Could you check a few things on this model? Use its own coordinates, in mm. Face numbers are marked on the shaded views. Round coordinates to 2 decimals unless told otherwise and drop trailing zeros. Loops run counter-clockwise (first coordinate to the right, second up) from the corner with the lowest first, then second, coordinate; pieces in that order, holes last. Notation, with made-up numbers: (13, 9.25) - (52, 9.25) arc R12 ccw to (52, 30.25) - close; hole circle Ø10 at (-26, -30.75). An arc over 180 degrees is marked (long way). Answer as CSV lines item,"result". Start each with the question number.
1) Suppose I cut it at C-C, the plane y = -25. Write out the boundary of the cut face in (x, z), then the cut area to 3 significant figures.
2) Suppose I cut it at A-A, the plane z = 7. Write out the boundary of the cut face in (x, y).
3) We'd pull the mould along X, two halves only. Please class the marked faces 1, 2, 3 and 4: pulls with the +X half, pulls with the -X half, needs draft (parallel to the pull), parting line crosses it, or undercut.
4) I'm going to push a flat-ended pin straight in: pin 1 Ø6 at (y, z) = (-19, 21.5) entering from -X. Where does the tip first touch, or does it pass through?
5) Suppose I cut it at D-D, the plane x = 16.25. Write out the boundary of the cut face in (y, z).
6) Please list where these lines run through material, in increasing order: line 1 along X through (y, z) = (-26.5, 10.25); line 2 along Z through (x, y) = (10.5, -19); line 3 along Y through (x, z) = (17.75, 10.25).
7) Suppose I cut it at B-B, the plane z = 17.25. Write out the boundary of the cut face in (x, y), then the cut area to 3 significant figures.
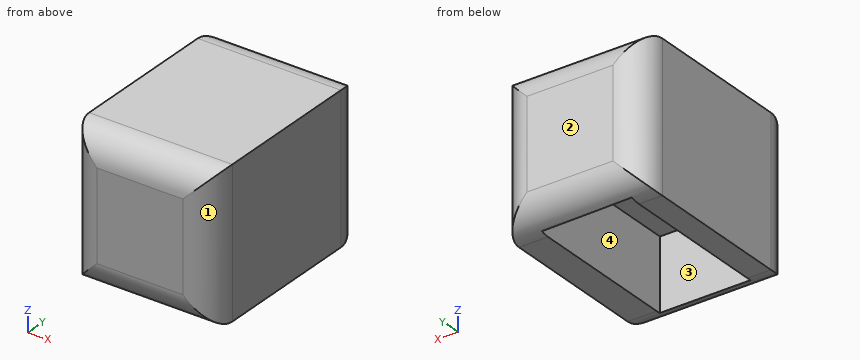
```python
from build123d import *

# Parameters (mm, degrees)
F0_W        = 36.6208925843
F0_H        = 25.9851198643
F1_DEPTH    = 25.4
F3_DEPTH    = 12.7
F4_DEPTH    = 12.7
F5_T1_DEPTH = 50.8
F5_T3_DEPTH = 51.3851198643
F6_T1_DEPTH = 50.8
F6_T3_DEPTH = 51.3851198643


# Not quite as in the source:
# - a fillet or chamfer that OpenCascade refuses, or shapes differently, is made with other operations: its cross-section is extruded or revolved along the edge and cut away or added


with BuildPart() as f1:
    # F0 (on Right) → F1 (new body)
    with BuildSketch(Plane.YZ):
        with Locations((-18.3104462922, 12.9925599322)):
            Rectangle(F0_W, F0_H)
    extrude(amount=F1_DEPTH)

    # F2 (on Top) → F3 (join)
    with BuildSketch(Plane.XY):
        Polygon((20.2587246895, -3.5579784308), (4.1429102421, -3.3661234193), (4.1429102421, -32.3362164199), (20.2587246895, -32.3362164199), align=None)
    extrude(amount=F3_DEPTH)

    # F2 (on Top) → F4 (cut)
    with BuildSketch(Plane.XY):
        Polygon((20.2587246895, -3.5579784308), (4.1429102421, -3.3661234193), (4.1429102421, -32.3362164199), (20.2587246895, -32.3362164199), align=None)
    extrude(amount=F4_DEPTH, mode=Mode.SUBTRACT)

    # F5: fillet of radius 5.08 on 4 edges, made by hand

    # F5_s2 → F5_t1 (cut)
    with BuildSketch(Plane.YZ.offset(-12.7)):
        with BuildLine():
            ThreePointArc((-36.6208925843, 20.9051198643), (-35.1329950328, 24.4972223128), (-31.5408925843, 25.9851198643))
            Line((-31.5408925843, 25.9851198643), (-36.6208925843, 25.9851198643))
            Line((-36.6208925843, 25.9851198643), (-36.6208925843, 20.9051198643))
        make_face()
        with BuildLine():
            ThreePointArc((-31.5408925843, 0), (-35.1329950328, 1.4878975516), (-36.6208925843, 5.08))
            Line((-36.6208925843, 5.08), (-36.6208925843, 0))
            Line((-36.6208925843, 0), (-31.5408925843, 0))
        make_face()
    extrude(amount=F5_T1_DEPTH, mode=Mode.SUBTRACT)

    # F5_s4 → F5_t3 (cut)
    with BuildSketch(Plane.XY.offset(-12.7)):
        with BuildLine():
            ThreePointArc((5.08, -36.6208925843), (1.4878975516, -35.1329950328), (0, -31.5408925843))
            Line((0, -31.5408925843), (0, -36.6208925843))
            Line((0, -36.6208925843), (5.08, -36.6208925843))
        make_face()
        with BuildLine():
            ThreePointArc((20.32, -36.6208925843), (23.9121024484, -35.1329950328), (25.4, -31.5408925843))
            Line((25.4, -31.5408925843), (25.4, -36.6208925843))
            Line((25.4, -36.6208925843), (20.32, -36.6208925843))
        make_face()
    extrude(amount=F5_T3_DEPTH, mode=Mode.SUBTRACT)

    # F6: fillet of radius 5.08 on 4 edges, made by hand

    # F6_s2 → F6_t1 (cut)
    with BuildSketch(Plane.YZ.offset(-12.7)):
        with BuildLine():
            ThreePointArc((-5.08, 0), (-1.4878975516, 1.4878975516), (0, 5.08))
            Line((0, 5.08), (0, 0))
            Line((0, 0), (-5.08, 0))
        make_face()
        with BuildLine():
            ThreePointArc((0, 20.9051198643), (-1.4878975516, 24.4972223128), (-5.08, 25.9851198643))
            Line((-5.08, 25.9851198643), (0, 25.9851198643))
            Line((0, 25.9851198643), (0, 20.9051198643))
        make_face()
    extrude(amount=F6_T1_DEPTH, mode=Mode.SUBTRACT)

    # F6_s4 → F6_t3 (cut)
    with BuildSketch(Plane.XY.offset(-12.7)):
        with BuildLine():
            ThreePointArc((0, -5.08), (1.4878975516, -1.4878975516), (5.08, 0))
            Line((5.08, 0), (0, 0))
            Line((0, 0), (0, -5.08))
        make_face()
        with BuildLine():
            ThreePointArc((20.32, 0), (23.9121024484, -1.4878975516), (25.4, -5.08))
            Line((25.4, -5.08), (25.4, 0))
            Line((25.4, 0), (20.32, 0))
        make_face()
    extrude(amount=F6_T3_DEPTH, mode=Mode.SUBTRACT)


solid = f1.part
```
Filled sheet:
1,outline,"(0, 0) - (4.14, 0) - (4.14, 12.7) - (20.26, 12.7) - (20.26, 0) - (25.4, 0) - (25.4, 25.99) - (0, 25.99) - close"
1,area,"455 mm²"
2,outline,"(0, -31.54) arc R5.08 ccw to (5.08, -36.62) - (20.32, -36.62) arc R5.08 ccw to (25.4, -31.54) - (25.4, -5.08) arc R5.08 ccw to (20.32, 0) - (5.08, 0) arc R5.08 ccw to (0, -5.08) - close; hole (4.14, -32.34) - (20.26, -32.34) - (20.26, -3.56) - (4.14, -3.37) - close"
3,face 1,"pulls with the +X half"
3,face 2,"needs draft"
3,face 3,"undercut"
3,face 4,"undercut"
4,pin 1,"x = 0"
5,outline,"(-36.62, 5.08) arc R5.08 ccw to (-32.34, 0.06) - (-32.34, 12.7) - (-3.51, 12.7) - (-3.51, 0.25) arc R5.08 ccw to (0, 5.08) - (0, 20.91) arc R5.08 ccw to (-5.08, 25.99) - (-31.54, 25.99) arc R5.08 ccw to (-36.62, 20.91) - close"
6,line 1,"0 to 4.14, 20.26 to 25.4"
6,line 2,"12.7 to 25.99"
6,line 3,"-36.62 to -32.34, -3.53 to 0"
7,outline,"(0, -31.54) arc R5.08 ccw to (5.08, -36.62) - (20.32, -36.62) arc R5.08 ccw to (25.4, -31.54) - (25.4, -5.08) arc R5.08 ccw to (20.32, 0) - (5.08, 0) arc R5.08 ccw to (0, -5.08) - close"
7,area,"908 mm²"
